Source: three-view drawing plus pictorial views. Frame: mm from the lowest corner of the part. A direction names the side the tool comes from. Coordinates: 2 decimals unless noted, no trailing zeros. Loops run counter-clockwise (first coordinate to the right, second up) from the corner with the lowest first, then second, coordinate; pieces in that order, holes last. Notation, with made-up numbers: M 32.25,76.25 L 75.25,76.25 A10 cw 75.25,93.25 Z; hole C 58.5,-14 d7. An arc over 180 degrees is marked long. Use a Markdown table: item, result. Add a question column.
1. Set-up query: the marked faces 4, 5 and 6. Return all of +Z, -Z, +X, -X, +Y, -Y with unobstructed straight access to the full face (end or side cutting, diameter ignored); none if empty.
2. Section B-B on x = 67.5. Output: boundary loops of the cut face in (y, z), then the cut area to 3 significant figures.
3. Section D-D on y = 26. Output: boundary loops of the cut face in (x, z), then the cut area to 3 significant figures.
4. Line query: L1, parallel to X at y = 3.5, z = 3.5; L2, parallel to Z at x = 54, y = 11; L3, parallel to Y at x = 56.5, z = 27. Output: solid intervals per line, ascending. Write a range as [from, to].
5. Pin query (flat end, axial travel): pin 1 (2.5 mm diameter, centred on y = 20.5, z = 3, fed in from -X); pin 2 (4 mm diameter, centred on y = 15, z = 28, fed in from -X); pin 3 (4 mm diameter, centred on x = 3.5, z = 37, fed in from +Y); pin 4 (6 mm diameter, centred on x = 9, z = 21.5, fed in from +Y). Return the tip coordinate at first contact, or that it passes through.
6. Section A-A on y = 5.5. Output: boundary loops of the cut face in (x, z), then the cut area to 3 significant figures.
7. Section C-C on z = 19.5. Output: boundary loops of the cut face in (x, y) (1 decimal).
8. Draft query along X for the marked faces 1, 2 and 3. Return one class per face: +X half, -X half, draft (parallel to the pull), parting line (faces both ways), or undercut.
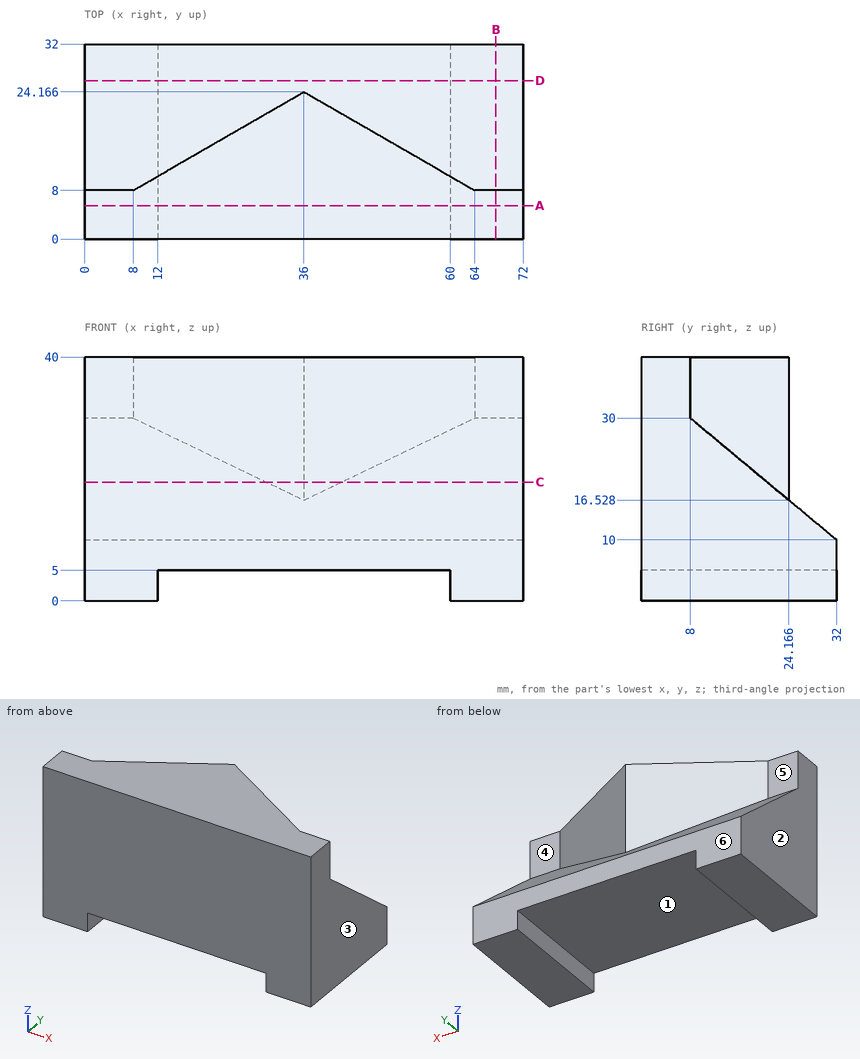
Answers below:
| question | item | result |
|---|---|---|
| 1 | face 4 | +Z, +X, +Y |
| 1 | face 5 | +Z, -X, +Y |
| 1 | face 6 | +Z, -Z, +X, -X, +Y |
| 2 | outline | M 0,0 L 32,0 L 32,10 L 8,30 L 8,40 L 0,40 Z |
| 2 | area | 800 mm² |
| 3 | outline | M 0,0 L 12,0 L 12,5 L 60,5 L 60,0 L 72,0 L 72,15 L 0,15 Z |
| 3 | area | 840 mm² |
| 4 | L1 | x = [0, 12], [60, 72] |
| 4 | L2 | z = [5, 40] |
| 4 | L3 | y = [0, 12.33] |
| 5 | pin 1 | stops at x = 0 |
| 5 | pin 2 | stops at x = 16.66 |
| 5 | pin 3 | stops at y = 8 |
| 5 | pin 4 | stops at y = 21.8 |
| 6 | outline | M 0,0 L 12,0 L 12,5 L 60,5 L 60,0 L 72,0 L 72,40 L 0,40 Z |
| 6 | area | 2,640 mm² |
| 7 | outline | M 0,0 L 72,0 L 72,20.6 L 42.2,20.6 L 36,24.2 L 29.8,20.6 L 0,20.6 Z |
| 8 | face 1 | undercut |
| 8 | face 2 | -X half |
| 8 | face 3 | +X half |
